The drawing under review shows one solid part. Ordinate dimensions are in mm from its lowest x, y, z. A direction names the side the tool comes from. Coordinates: 2 decimals unless noted, no trailing zeros. Loops run counter-clockwise (first coordinate to the right, second up) from the corner with the lowest first, then second, coordinate; pieces in that order, holes last. Notation, with made-up numbers: M -3.75,37.5 L 8.25,37.5 A26 cw 8.25,68.5 Z; hole C -8,0 d3. An arc over 180 degrees is marked long. Return JSON: item names as keys, results as strings.
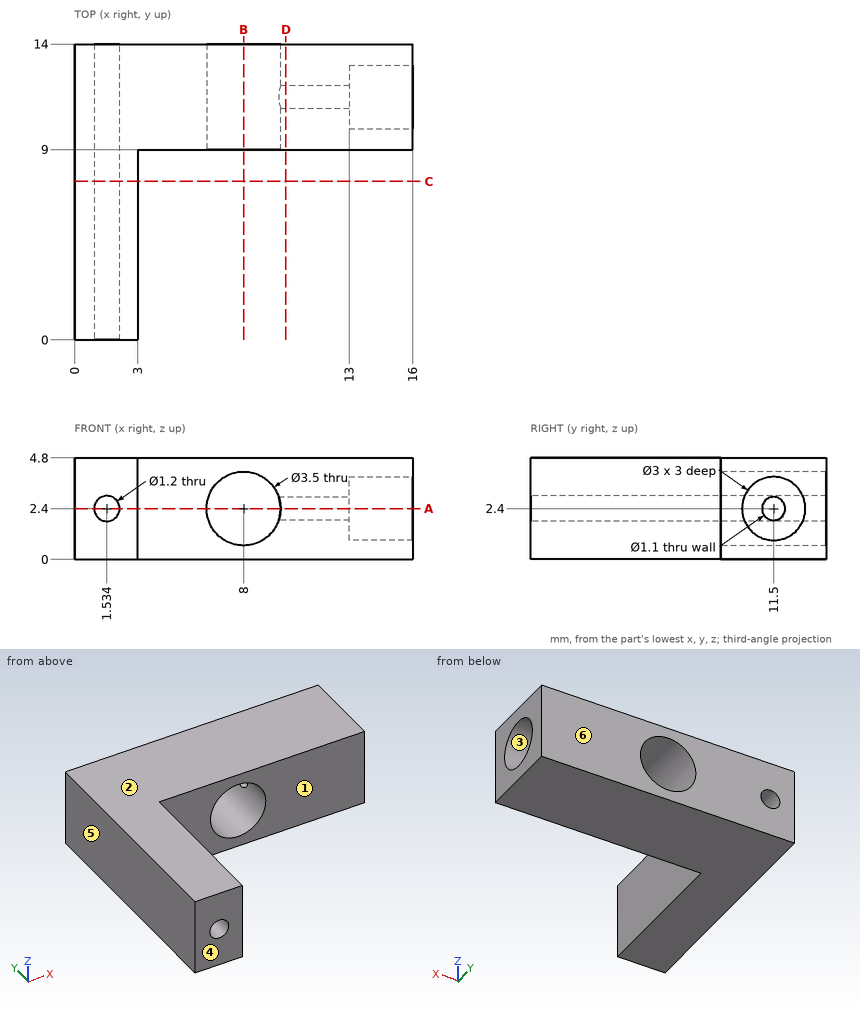
1. Add section D-D on x = 10. Give the boundary of the cut face in (y, z).
Check values:
{"outline": "M 9,0 L 14,0 L 14,4.8 L 9,4.8 Z; hole C 11.5,2.4 d1.1"}
2. The part is to be moulded in two halves that separate along Y. For the marked faces 3, 4, 5 and 6, say which applies: released by +Y, released by -Y, zero draft, split by the parting line, or undercut.
Check values:
{"face 3": "undercut", "face 4": "released by -Y", "face 5": "zero draft", "face 6": "released by +Y"}
3. Add section B-B on x = 8. Give the boundary of the cut face in (y, z).
Check values:
{"outline": "M 9,0 L 14,0 L 14,0.65 L 9,0.65 Z; M 9,4.15 L 14,4.15 L 14,4.8 L 9,4.8 Z"}
4. To check wall thickness, follow line 1 (Z direction, x = 11.75, y = 11.5); line 2 (Y direction, x = 4.25, z = 3.8); line 3 (X direction, y = 2, z = 4.45). State the ranges of each line that lie inside material, in increasing order.
Check values:
{"line 1": "0 to 1.85, 2.95 to 4.8", "line 2": "9 to 14", "line 3": "0 to 3"}
5. Machinability: for the marked faces 1 and 2, which of the approach directions +Z, -Z, +X, -X, +Y, -Y give a long, thin tool a straight path to every point of the face, cutting with its end or side? Answer none if there is none.
Check values:
{"face 1": "+Z, -Z, +X, -Y", "face 2": "+Z, +X, -X, +Y, -Y"}
6. Add section A-A on z = 2.4. Give the boundary of the cut face in (x, y), plus the area to 3 significant figures.
Check values:
{"outline": "M 0,0 L 0.93,0 L 0.93,14 L 0,14 Z; M 2.13,0 L 3,0 L 3,9 L 6.25,9 L 6.25,14 L 2.13,14 Z; M 9.75,9 L 16,9 L 16,10 L 13,10 L 13,10.95 L 9.75,10.95 Z; M 9.75,12.05 L 13,12.05 L 13,13 L 16,13 L 16,14 L 9.75,14 Z", "area": "60.1 mm²"}
7. Insertion check: pin 1 Ø1 at (x, z) = (12.5, 3.5) entering from -Y; pin 2 Ø2.5 at (y, z) = (4, 2.5) entering from +X; pin 3 Ø1.5 at (x, y) = (5.5, 2.5) entering from +Z. Each pin has a flat end and moves straight along its axis. Give the tip position at first contact, or say it passes through.
Check values:
{"pin 1": "y = 9", "pin 2": "x = 3", "pin 3": "through"}
8. Add section C-C on y = 7.5. Give the boundary of the cut face in (x, z), plus the area to 3 significant figures.
Check values:
{"outline": "M 0,0 L 3,0 L 3,4.8 L 0,4.8 Z; hole C 1.53,2.4 d1.2", "area": "13.3 mm²"}
